Geometry check sheet. Reference: the model listing, model coordinates, mm. A direction names the side the tool comes from. Coordinates: 2 decimals unless noted, no trailing zeros. Order: outer loops, then holes, each group sorted by start corner. A loop starts at its lowest first (then second) coordinate and runs counter-clockwise, first axis right, second up.
```python
from build123d import *

# Parameters (mm, degrees)
F1_DEPTH = 25.4
F3_DEPTH = 25.4
F5_DEPTH = 25.4
F6_R     = 6.35
F7_DEPTH = 25.4
F9_DEPTH = 25.4


with BuildPart() as f1:
    # F0 (on Front) → F1 (new body)
    with BuildSketch(Plane.XZ):
        Polygon((-31.75, 38.1), (-57.15, 38.1), (-57.15, 0), (0, 0), (0, 12.7), (-31.75, 12.7), align=None)
    extrude(amount=F1_DEPTH)

    # F2 (on face) → F3 (cut)
    with BuildSketch(Plane.YZ.offset(-31.75)):
        with BuildLine():
            Line((-6.35, 38.1), (-19.05, 38.1))
            add(Edge.make_bspline(
                [(-19.05, 38.1), (-18.5709856451, 19.3447768688), (-6.809361279, 18.4162277728), (-6.35, 38.1)],
                knots=[0, 0, 0, 0, 12.7, 12.7, 12.7, 12.7], degree=3))
        make_face()
    extrude(amount=-F3_DEPTH, mode=Mode.SUBTRACT)

    # F4 (on face) → F5 (cut)
    with BuildSketch(Plane.XY.offset(12.7)):
        with BuildLine():
            Line((0, -25.4), (0, -12.7))
            ThreePointArc((0, -12.7), (-4.6286120427, -20.7713879573), (-12.7, -25.4))
            Line((-12.7, -25.4), (0, -25.4))
        make_face()
        with BuildLine():
            ThreePointArc((-15.875, 0), (-5.8860880189, -3.7857350236), (0, -12.7))
            Line((0, -12.7), (0, 0))
            Line((0, 0), (-15.875, 0))
        make_face()
    extrude(amount=-F5_DEPTH, mode=Mode.SUBTRACT)

    # F6 (on face) → F7 (cut)
    with BuildSketch(Plane.XY.offset(12.7)):
        with Locations((-23.5232505947, -12.8449322656)):
            Circle(F6_R)
        with Locations((-8.7082285261, -12.0423395505)):
            Circle(F6_R)
    extrude(amount=-F7_DEPTH, mode=Mode.SUBTRACT)

    # F8 (on face) → F9 (cut)
    with BuildSketch(Plane(origin=(-57.15, 0, 0), x_dir=(0, -1, 0), z_dir=(-1, 0, 0))):
        with BuildLine():
            Line((25.4, 38.1), (19.05, 38.1))
            ThreePointArc((19.05, 38.1), (23.5401280605, 36.2401280605), (25.4, 31.75))
            Line((25.4, 31.75), (25.4, 38.1))
        make_face()
        with BuildLine():
            ThreePointArc((0, 31.75), (1.8598719395, 36.2401280605), (6.35, 38.1))
            Line((6.35, 38.1), (0, 38.1))
            Line((0, 38.1), (0, 31.75))
        make_face()
    extrude(amount=-F9_DEPTH, mode=Mode.SUBTRACT)


solid = f1.part
```
Item 1: Sectioned sample at B-B (z = 4). Record the cut outline in (x, y) (3 decimals), and give its area (3 significant figures).
Item 2: Release check for a two-part mould opening along Y. For faces 3 (the face through (-2.651, -10.135, 6.439)), 4 (the face through (-57.15, -13, 15)), 5 (the face through (-44.63, -23.49, 36.29)) record: pulls with the +Y half, pulls with the -Y half, needs draft (parallel to the pull), parting line crosses it, or undercut.
Item 3: Sectioned sample at A-A (x = -4). Record the cut outline in (y, z), and give its area (3 significant figures).
Item 4: Sectioned sample at C-C (y = -10.75). Give the number of separate pieces and of enclosed holes in the cut face, and give its area (3 significant figures).
Item 5: Depth check by flat-ended pin: P1, Ø7.5, axis at x = -10, y = -7.5, coming from the +Z side; P2, Ø1.5, axis at x = -28, y = -10, coming from the -Z side; P3, Ø10, axis at y = -22, z = 24.5, coming from the +X side. Enter the tip coordinate at first touch or a pass-through.
Item 6: Tool access check on faces 1 (the face through (-31.75, -13, 22)), 2 (the face through (-44.63, -1.81, 36.19)). Record the directions out of +Z, -Z, +X, -X, +Y, -Y that give a thin tool (end or side, any length) a straight path to the whole face; none if there is none.
Item 7: Sectioned sample at D-D (z = 15.5). Record the cut outline in (x, y).
Item 8: Thickness scan on line 1 along X through (y, z) = (-17.25, 7); line 2 along X through (y, z) = (-7.5, 2); line 3 along Y through (x, z) = (-53, 25). Record the ranges inside material, lowest first.
Geometry check:
1. outline: (-57.15, -25.4) - (-12.7, -25.4) arc R17.781 ccw to (0, -12.7) arc R17.374 ccw to (-15.875, 0) - (-57.15, 0) - close; hole circle Ø12.7 at (-23.523, -12.845); hole circle Ø12.7 at (-8.708, -12.042)
1. area: 1,090 mm2
2. face 3: undercut
2. face 4: needs draft
2. face 5: pulls with the -Y half
3. outline: (-20.11, 0) - (-16.3, 0) - (-16.3, 12.7) - (-20.11, 12.7) - close; (-7.78, 0) - (-5.54, 0) - (-5.54, 12.7) - (-7.78, 12.7) - close
3. area: 76.8 mm2
4. separate pieces: 3
4. enclosed holes: 0
4. area: 701 mm2
5. P1: stops at z = 12.7
5. P2: passes through
5. P3: stops at x = -31.75
6. face 1: +Z, +X, +Y, -Y
6. face 2: +Z, +X, -X, +Y
7. outline: (-57.15, -25.4) - (-31.75, -25.4) - (-31.75, 0) - (-57.15, 0) - close
8. line 1: x = -57.15 to -28.1, -18.95 to -12.34, -5.07 to -1.9
8. line 2: x = -57.15 to -26.95, -20.09 to -13.15, -4.27 to -2.43
8. line 3: y = -25.4 to -15.29, -9.91 to 0
